Work out the finished part from the listing and answer in its coordinate system (mm). Coordinates: 2 decimals unless noted, no trailing zeros. Order: outer loops, then holes, each group sorted by start corner. A loop starts at its lowest first (then second) coordinate and runs counter-clockwise, first axis right, second up. Notation, with made-up numbers: (52, 49) - (56, 49) arc R15 ccw to (56, 71) - close; hole circle Ø6 at (83.5, 5). An arc over 180 degrees is marked (long way). Answer as a JSON object with one key per item and string values. Group by question number.
1) Section A-A (x = -42) is taken. Give the vertices of the cut face in (y, z), plus the area to 3 significant figures.
2) Find the intervals of material crossed by line 1 along Z through (x, y) = (-24, 5.35); line 2 along Z through (x, y) = (-32, 1.2); line 3 along Z through (x, y) = (-69, 2.2), in increasing order.
3) Each of these flat-tipped pins is pushed along its axis until it touches: P1, Ø3.5, axis at y = 4.5, z = -154, coming from the +X side; P2, Ø1, axis at x = -101.5, y = 4.5, coming from the -Z side; P3, Ø1.8, axis at y = 4.5, z = -3, coming from the +X side; P4, Ø1.8, axis at x = -35, y = 4, coming from the +Z side. Where does it stop, or does it pass through?
4) Section B-B (y = 3.5) is taken. Count the separate pieces of the cut face and the enclosed holes in it, plus the area to 3 significant figures.
from build123d import *

# Parameters (mm, degrees)
ESQUISSE1_W             = 15
ESQUISSE1_H             = 6
BOSS_EXTRU_1_DEPTH      = 6
ESQUISSE2_W             = 15
ESQUISSE2_H             = 3
ENL_V_MAT_EXTRU_1_DEPTH = 6


with BuildPart() as part:
    # Esquisse1 → Boss.-Extru.1 (new body)
    with BuildSketch(Plane(origin=(0, 0, 0), x_dir=(1, 0, 0), z_dir=(0, 1, 0))):
        with Locations((-122.5, 273)):
            Rectangle(ESQUISSE1_W, ESQUISSE1_H)
        with Locations((-87.5, 273)):
            Rectangle(ESQUISSE1_W, ESQUISSE1_H)
        with Locations((-52.5, 273)):
            Rectangle(ESQUISSE1_W, ESQUISSE1_H)
        with Locations((-17.5, 273)):
            Rectangle(ESQUISSE1_W, ESQUISSE1_H)
        Polygon((-140, 270), (-140, 138), (0, 138), (0, 270), (-10, 270), (-25, 270), (-45, 270), (-60, 270), (-80, 270), (-95, 270), (-115, 270), (-130, 270), align=None)
        Polygon((0, 138), (-140, 138), (-140, 6), (-130, 6), (-115, 6), (-95, 6), (-80, 6), (-60, 6), (-45, 6), (-25, 6), (-10, 6), (0, 6), align=None)
        with Locations((-122.5, 3)):
            Rectangle(ESQUISSE1_W, ESQUISSE1_H)
        with Locations((-87.5, 3)):
            Rectangle(ESQUISSE1_W, ESQUISSE1_H)
        with Locations((-52.5, 3)):
            Rectangle(ESQUISSE1_W, ESQUISSE1_H)
        with Locations((-17.5, 3)):
            Rectangle(ESQUISSE1_W, ESQUISSE1_H)
    extrude(amount=BOSS_EXTRU_1_DEPTH)

    # Esquisse2 → Enlèv. mat.-Extru.1 (cut)
    with BuildSketch(Plane.XZ):
        with Locations((-1.5, -154.5)):
            Rectangle(ESQUISSE2_W, ESQUISSE2_H)
        with Locations((-28.5, -154.5)):
            Rectangle(ESQUISSE2_W, ESQUISSE2_H)
        with Locations((-55.5, -154.5)):
            Rectangle(ESQUISSE2_W, ESQUISSE2_H)
        with Locations((-82.5, -154.5)):
            Rectangle(ESQUISSE2_W, ESQUISSE2_H)
        with Locations((-109.5, -154.5)):
            Rectangle(ESQUISSE2_W, ESQUISSE2_H)
        with Locations((-136.5, -154.5)):
            Rectangle(ESQUISSE2_W, ESQUISSE2_H)
    extrude(amount=-ENL_V_MAT_EXTRU_1_DEPTH, mode=Mode.SUBTRACT)


solid = part.part
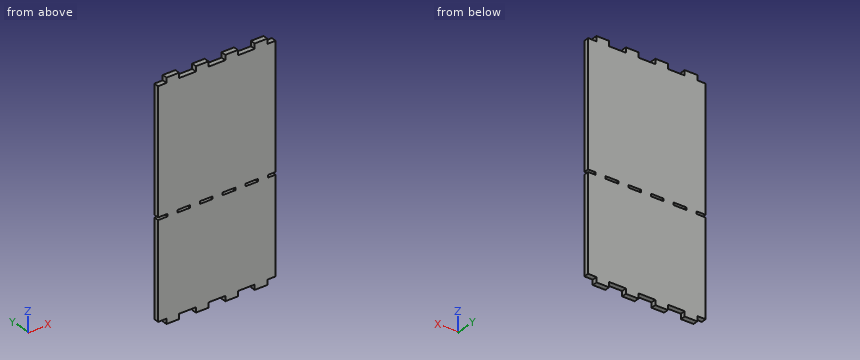
Report:
{
 "1": {"outline": "(0, -270) - (6, -270) - (6, -6) - (0, -6) - close", "area": "1,580 mm²"},
 "2": {"line 1": "z = -276 to -156, -153 to 0", "line 2": "z = -270 to -156, -153 to -6", "line 3": "z = -270 to -6"},
 "3": {"P1": "stops at x = 0", "P2": "stops at z = -270", "P3": "stops at x = -10", "P4": "stops at z = -6"},
 "4": {"separate pieces": "1", "enclosed holes": "4", "area": "37,400 mm²"}
}
